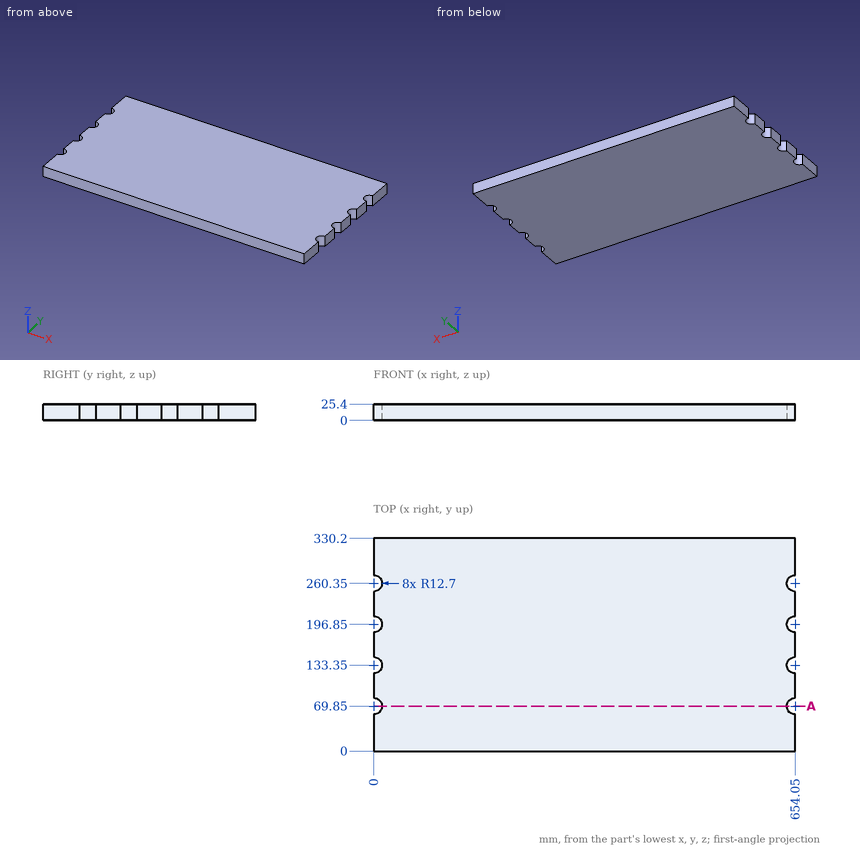
Could you check a few things on this drawing? It's one solid part, dimensions in mm from its lowest x, y, z. Round coordinates to 2 decimals unless told otherwise and drop trailing zeros. Order: outer loops, then holes, each group sorted by start corner. A loop starts at its lowest first (then second) coordinate and runs counter-clockwise, first axis right, second up.
Q1. I'm going to push a flat-ended pin straight in: P1, Ø1, axis at y = 267.5, z = 6, coming from the +X side. Where does the tip first touch, or does it pass through?
Geometry says:
P1: stops at x = 643.91
Q2. Imagine slicing it at A-A, the plane y = 69.85. List the corners of the cut face in (x, z) for me, then the cut area to 3 significant figures.
Geometry says:
outline: (12.7, 0) - (641.35, 0) - (641.35, 25.4) - (12.7, 25.4) - close
area: 16,000 mm2
Q3. Please list where these lines run through material, in increasing order: probe 1 along X at (y, z) = (134.5, 3.75); probe 2 along X at (y, z) = (69, 16).
Geometry says:
probe 1: x = 12.65 to 641.4
probe 2: x = 12.67 to 641.38
